from build123d import *

# Parameters (mm, degrees)
SKETCH1_W             = 12.75
SKETCH1_H             = 6
BOSS_EXTRUDE1_DEPTH   = 6
F_1_0MM_DOWEL_HOLE1_D = 1.75
SKETCH4_W             = 1
SKETCH4_H             = 2.5
BOSS_EXTRUDE2_DEPTH   = 0.5
SKETCH7_W             = 0.4
SKETCH7_H             = 0.4
EXTRUDE_THIN6_DEPTH   = 2
FILLET9_R             = 0.2


with BuildPart() as part:
    # Sketch1 → Boss-Extrude1 (new body)
    with BuildSketch(Plane.XY):
        with Locations((6.375, 3)):
            Rectangle(SKETCH1_W, SKETCH1_H)
    extrude(amount=BOSS_EXTRUDE1_DEPTH)

    # Ø1.0mm Dowel Hole1 (through all)
    with Locations(Plane.XY.offset(6)):
        with Locations((3.375, 1.15), (9.375, 1.15)):
            Hole(F_1_0MM_DOWEL_HOLE1_D / 2)

    # Sketch4 → Boss-Extrude2 (add)
    with BuildSketch(Plane(origin=(0, 6, 0), x_dir=(1, 0, 0), z_dir=(0, 1, 0))):
        with Locations((4, -3)):
            Rectangle(SKETCH4_W, SKETCH4_H)
    extrude(amount=BOSS_EXTRUDE2_DEPTH)

    # Sketch7 → Extrude-Thin6 (add)
    with BuildSketch(Plane.XZ):
        with Locations((11.5, 3)):
            Rectangle(SKETCH7_W, SKETCH7_H)
        with Locations((6.375, 3)):
            Rectangle(SKETCH7_W, SKETCH7_H)
        with Locations((1.25, 3)):
            Rectangle(SKETCH7_W, SKETCH7_H)
    extrude(amount=EXTRUDE_THIN6_DEPTH)

    # Fillet9
    fillet9_edges = [part.edges().sort_by_distance(p)[0] for p in [
        (6.575, -2, 3),
        (6.375, -2, 3.2),
        (6.175, -2, 3),
        (6.375, -2, 2.8),
        (1.45, -2, 3),
        (1.25, -2, 3.2),
        (1.05, -2, 3),
        (1.25, -2, 2.8),
        (11.3, -2, 3),
        (11.5, -2, 2.8),
        (11.7, -2, 3),
        (11.5, -2, 3.2),
    ]]
    fillet(fillet9_edges, radius=FILLET9_R - 0.0001)  # a hair under: the kernel refuses the full size


solid = part.part
Read the model definition and answer for the solid it produces. Units are mm, in the model's axes. Coordinates: 2 decimals unless noted, no trailing zeros. Loops run counter-clockwise (first coordinate to the right, second up) from the corner with the lowest first, then second, coordinate; pieces in that order, holes last. Notation, with made-up numbers: (55.25, -4.75) -> (99.25, -4.75) arc R7 ccw to (99.25, 4.25) -> close; hole circle Ø9 at (42, 43). An arc over 180 degrees is marked (long way). Answer in a Markdown table with one row per item.
Item 1: A cutting plane is placed at C-C on x = 3.25. Determine the outline of the cut face in (y, z), plus the area to 3 significant figures.
Returned:
| item | result |
|---|---|
| outline | (0, 0) -> (0.28, 0) -> (0.28, 6) -> (0, 6) -> close; (2.02, 0) -> (6, 0) -> (6, 6) -> (2.02, 6) -> close |
| area | 25.6 mm^2 |
Item 2: A cutting plane is placed at D-D on y = -1. Determine the outline of the cut face in (x, z) (3 decimals), plus the area to 3 significant figures.
Returned:
| item | result |
|---|---|
| outline | (1.05, 2.8) -> (1.45, 2.8) -> (1.45, 3.2) -> (1.05, 3.2) -> close; (6.175, 2.8) -> (6.575, 2.8) -> (6.575, 3.2) -> (6.175, 3.2) -> close; (11.3, 2.8) -> (11.7, 2.8) -> (11.7, 3.2) -> (11.3, 3.2) -> close |
| area | 0.480 mm^2 |
Item 3: Straight lines are drawn through the part: line 1 along Y through (x, z) = (5.5, 1.55); line 2 along X through (y, z) = (1.5, 5.4); line 3 along Y through (x, z) = (3, 4.25). For each, find the intervals that lie inside material, in ascending order. Write a range as [from, to].
Returned:
| item | result |
|---|---|
| line 1 | y = [0, 6] |
| line 2 | x = [0, 2.57], [4.18, 8.57], [10.18, 12.75] |
| line 3 | y = [0, 0.36], [1.94, 6] |
Item 4: A cutting plane is placed at A-A on y = 1.15. Determine the outline of the cut face in (x, z), plus the area to 3 significant figures.
Returned:
| item | result |
|---|---|
| outline | (0, 0) -> (2.5, 0) -> (2.5, 6) -> (0, 6) -> close; (4.25, 0) -> (8.5, 0) -> (8.5, 6) -> (4.25, 6) -> close; (10.25, 0) -> (12.75, 0) -> (12.75, 6) -> (10.25, 6) -> close |
| area | 55.5 mm^2 |
Item 5: A cutting plane is placed at B-B on z = 1.95. Determine the outline of the cut face in (x, y) (3 decimals).
Returned:
| item | result |
|---|---|
| outline | (0, 0) -> (12.75, 0) -> (12.75, 6) -> (4.5, 6) -> (4.5, 6.5) -> (3.5, 6.5) -> (3.5, 6) -> (0, 6) -> close; hole circle Ø1.75 at (3.375, 1.15); hole circle Ø1.75 at (9.375, 1.15) |
Item 6: Each of these flat-tipped pins is pushed along its axis until it touches: P1, Ø3, axis at x = 4, z = 4.5, coming from the -Y side; P2, Ø2, axis at x = 9.5, z = 2, coming from the +Y side. Where does it stop, or does it pass through?
Returned:
| item | result |
|---|---|
| P1 | stops at y = 0 |
| P2 | stops at y = 6 |
Item 7: For a pull along X with two mould halves and no side action, classify faces 1 (the flat face through (6, 6, 3)), 2 (the flat face through (0, 3, 3)), 3 (the cylindrical face through (10.07, 0.62, 2.96)) as released by +X, released by -X, zero draft, split by the parting line, or undercut.
Returned:
| item | result |
|---|---|
| face 1 | zero draft |
| face 2 | released by -X |
| face 3 | undercut |
